from build123d import *

# Parameters (mm, degrees)
STIRNSENKUNG_F_R_M4_ZYLINDERSCHRAUBE_MIT_D           = 4.3
STIRNSENKUNG_F_R_M4_ZYLINDERSCHRAUBE_MIT_CBORE_D     = 8
STIRNSENKUNG_F_R_M4_ZYLINDERSCHRAUBE_MIT_CBORE_DEPTH = 2
FASE1_SIZE                                           = 1
FASE2_SIZE                                           = 0.5


with BuildPart() as part:
    # Skizze1 → Rotation1 (revolve)
    with BuildSketch(Plane.XY):
        Polygon((0, 0), (0, 25), (-4, 25), (-4, 5), (-6, 5), (-6, 0), align=None)
    revolve(axis=Axis((0, 0, 0), (0, -1, 0)))

    # Stirnsenkung für M4 Zylinderschraube mit Innensechskant1 (through all)
    with Locations(Plane(origin=(0, 0, 0), x_dir=(-1, 0, 0), z_dir=(0, -1, 0))):
        with Locations((0, 0)):
            CounterBoreHole(STIRNSENKUNG_F_R_M4_ZYLINDERSCHRAUBE_MIT_D / 2, STIRNSENKUNG_F_R_M4_ZYLINDERSCHRAUBE_MIT_CBORE_D / 2, STIRNSENKUNG_F_R_M4_ZYLINDERSCHRAUBE_MIT_CBORE_DEPTH)

    # Fase1
    fase1_edges = [part.edges().sort_by_distance(p)[0] for p in [
        (6, 0, 0),
        (6, 5, 0),
    ]]
    chamfer(fase1_edges, length=FASE1_SIZE)

    # Fase2
    fase2_edges = [part.edges().sort_by_distance(p)[0] for p in [
        (4, 25, 0),
    ]]
    chamfer(fase2_edges, length=FASE2_SIZE)


solid = part.part
The listing builds one solid part. Answer for the finished solid, in the listing's coordinates (mm). A direction names the side the tool comes from. Give positions to 0.01 mm unless a question says otherwise; leave off trailing zeros. Loops run counter-clockwise (first coordinate to the right, second up) from the corner with the lowest first, then second, coordinate; pieces in that order, holes last.
Item 1: Determine the mould class of faces 1 (the cylindrical face through (-2.15, 13.66, -0.09)), 2 (the cylindrical face through (0.867, 14.614, 3.905)), 3 (the flat face through (-2, 25, 2)) for opening direction Z: +Z half, -Z half, draft (parallel to the pull), parting line (faces both ways), or undercut.
Derived:
face 1: undercut
face 2: parting line
face 3: draft
Item 2: A cutting plane is placed at C-C (y = 3.25). Give the vertices of the cut face in (x, z), then the cut area to 3 significant figures.
Derived:
outline: circle Ø12 at (0, 0); hole circle Ø4.3 at (0, 0)
area: 98.6 mm2
Item 3: Each of these flat-tipped pins is pushed along its axis until it touches: pin 1 Ø5 at (x, y) = (-3, 16) entering from +Z; pin 2 Ø1.5 at (x, y) = (-4, 21.5) entering from +Z; pin 3 Ø1 at (x, y) = (-2.5, 13.5) entering from +Z; pin 4 Ø4 at (x, z) = (2, 4) entering from +Y. Where does it stop, or does it pass through?
Derived:
pin 1: stops at z = 3.97
pin 2: stops at z = 2.33
pin 3: stops at z = 3.46
pin 4: stops at y = 25
Item 4: A cutting plane is placed at B-B (z = 0). Give the vertices of the cut face in (x, y).
Derived:
outline: (-6, 1) - (-5, 0) - (-4, 0) - (-4, 2) - (-2.15, 2) - (-2.15, 25) - (-3.5, 25) - (-4, 24.5) - (-4, 5) - (-5, 5) - (-6, 4) - close; (2.15, 2) - (4, 2) - (4, 0) - (5, 0) - (6, 1) - (6, 4) - (5, 5) - (4, 5) - (4, 24.5) - (3.5, 25) - (2.15, 25) - close
Item 5: A tool of negligible diameter and unlimited length cuts with its end or side. For faces 4 (the cylindrical face through (6, 2, 0)), 5 (the cylindrical face through (0.867, 0.986, 3.905)), from which of +Z, -Z, +X, -X, +Y, -Y can it reach the whole face along a straight path? Write none if from no direction.
Derived:
face 4: +Y, -Y
face 5: -Y
Item 6: A cutting plane is placed at A-A (x = 0). Give the vertices of the cut face in (y, z).
Derived:
outline: (0, -5) - (1, -6) - (4, -6) - (5, -5) - (5, -4) - (24.5, -4) - (25, -3.5) - (25, -2.15) - (2, -2.15) - (2, -4) - (0, -4) - close; (0, 4) - (2, 4) - (2, 2.15) - (25, 2.15) - (25, 3.5) - (24.5, 4) - (5, 4) - (5, 5) - (4, 6) - (1, 6) - (0, 5) - close
Item 7: A cutting plane is placed at D-D (y = 23). Give the vertices of the cut face in (x, z), then the cut area to 3 significant figures.
Derived:
outline: circle Ø8 at (0, 0); hole circle Ø4.3 at (0, 0)
area: 35.7 mm2
Item 8: Find the intervals of material crossed by line 1 along Z through (x, y) = (0, 16.25); line 2 along Y through (x, z) = (0.5, -4.5); line 3 along X through (y, z) = (17.25, 0.75), in increasing order.
Derived:
line 1: z = -4 to -2.15, 2.15 to 4
line 2: y = 0 to 5
line 3: x = -3.93 to -2.01, 2.01 to 3.93
